from build123d import *

# Parameters (mm, degrees)
F1_DEPTH = 5
F3_DEPTH = 5.001


with BuildPart() as f1:
    # F0 (on Front) → F1 (new body)
    with BuildSketch(Plane.XZ):
        Polygon((-267.89507, 257.257965), (-455.89507, 257.257965), (-455.89507, -187.742035), (-307.39507, -187.742035), (-307.39507, -122.742035), (-267.89507, -122.742035), align=None)
    extrude(amount=F1_DEPTH)

    # F2 (on face) → F3 (cut, through all)
    with BuildSketch(Plane.XZ.offset(5)):
        with BuildLine():
            ThreePointArc((-378.89507, 81.257965), (-421.321476, 63.684372), (-438.89507, 21.257965))
            ThreePointArc((-438.89507, 21.257965), (-378.89507, -38.742035), (-318.89507, 21.257965))
            ThreePointArc((-318.89507, 21.257965), (-336.468663, 63.684372), (-378.89507, 81.257965))
        make_face()
        with BuildLine():
            ThreePointArc((-318.89507, 147.257965), (-336.468663, 189.684372), (-378.89507, 207.257965))
            Line((-378.89507, 207.257965), (-378.89507, 147.257965))
            Line((-378.89507, 147.257965), (-378.89507, 87.257965))
            ThreePointArc((-378.89507, 87.257965), (-336.468663, 104.831558), (-318.89507, 147.257965))
        make_face()
        with BuildLine():
            Line((-378.89507, 147.257965), (-438.89507, 147.257965))
            ThreePointArc((-438.89507, 147.257965), (-421.321477, 104.831558), (-378.89507, 87.257965))
            Line((-378.89507, 87.257965), (-378.89507, 147.257965))
        make_face()
        with BuildLine():
            Line((-378.89507, 147.257965), (-378.89507, 207.257965))
            ThreePointArc((-378.89507, 207.257965), (-421.321477, 189.684372), (-438.89507, 147.257965))
            Line((-438.89507, 147.257965), (-378.89507, 147.257965))
        make_face()
    extrude(amount=-F3_DEPTH, mode=Mode.SUBTRACT)


solid = f1.part
Can you work these out from the model? Positions are in its coordinate system, mm. Coordinates: 2 decimals unless noted, no trailing zeros. Loops run counter-clockwise (first coordinate to the right, second up) from the corner with the lowest first, then second, coordinate; pieces in that order, holes last. Notation, with made-up numbers: (5, 21) - (55, 21) arc R16 ccw to (55, 46) - close; hole circle Ø7 at (15.25, 78.25). An arc over 180 degrees is marked (long way). Put each result on its own line as item: value. Start each with the question number.
Item 1: Suppose I cut it at D-D (x = -416.5). Please give me the cut outline in (y, z), and give its area (3 significant figures).
Item 2: Suppose I cut it at A-A (y = -4.1). Please give me the cut outline in (x, z), and give its area (3 significant figures).
Item 3: If I drill on line 1 along Z through (x, y) = (-381, -0.55); line 2 along Z through (x, y) = (-373, -2.75); line 3 along X through (y, z) = (-2.35, 42.5), over which ranges is the centre line in solid material (lowest first)?
Item 4: Suppose I cut it at B-B (x = -389.5). Please give me the cut outline in (y, z).
Item 5: Suppose I cut it at C-C (z = 16). Please give me the cut outline in (x, y).
Here are the results:
1. outline: (-5, -187.74) - (0, -187.74) - (0, -25.5) - (-5, -25.5) - close; (-5, 68.01) - (0, 68.01) - (0, 100.5) - (-5, 100.5) - close; (-5, 194.01) - (0, 194.01) - (0, 257.26) - (-5, 257.26) - close
1. area: 1,290 mm²
2. outline: (-455.9, -187.74) - (-307.4, -187.74) - (-307.4, -122.74) - (-267.9, -122.74) - (-267.9, 257.26) - (-455.9, 257.26) - close; hole (-438.9, 21.26) arc R60 ccw (long way) to (-378.9, 81.26) arc R60 ccw to start; hole circle Ø120 at (-378.9, 147.26)
2. area: 58,500 mm²
3. line 1: -187.74 to -38.71, 81.22 to 87.29, 207.22 to 257.26
3. line 2: -187.74 to -38.45, 80.97 to 87.55, 206.97 to 257.26
3. line 3: -455.9 to -435.01, -322.78 to -267.9
4. outline: (-5, -187.74) - (0, -187.74) - (0, -37.8) - (-5, -37.8) - close; (-5, 80.31) - (0, 80.31) - (0, 88.2) - (-5, 88.2) - close; (-5, 206.31) - (0, 206.31) - (0, 257.26) - (-5, 257.26) - close
5. outline: (-455.9, -5) - (-438.66, -5) - (-438.66, 0) - (-455.9, 0) - close; (-319.13, -5) - (-267.9, -5) - (-267.9, 0) - (-319.13, 0) - close
